The listing builds one solid part. Answer for the finished solid, in the listing's coordinates (mm). A direction names the side the tool comes from. Coordinates: 2 decimals unless noted, no trailing zeros. Loops run counter-clockwise (first coordinate to the right, second up) from the corner with the lowest first, then second, coordinate; pieces in that order, holes last. Notation, with made-up numbers: (-1, 73.25) -> (8, 73.25) arc R11 ccw to (8, 94.25) -> close; hole circle Ø5 at (2.5, 80.25). An arc over 180 degrees is marked (long way). Answer in a Markdown table with one row per item.
```python
from build123d import *

# Parameters (mm, degrees)
F0_W      = 24
F0_H      = 24
F1_DEPTH  = 9.5
F4_R      = 4
F7_DEPTH  = 9.501
F8_DEPTH  = 4.5
F9_DEPTH  = 3.5
F5_R      = 1.35
F10_DEPTH = 9.501


with BuildPart() as f1:
    # F0 (on Top) → F1 (new body)
    with BuildSketch(Plane.XY):
        with Locations((12, 12)):
            Rectangle(F0_W, F0_H)
    extrude(amount=F1_DEPTH)

    # F4
    f4_edges = [f1.edges().sort_by_distance(p)[0] for p in [
        (0, 0, 4.75),
        (24, 0, 4.75),
        (24, 24, 4.75),
        (0, 24, 4.75),
    ]]
    fillet(f4_edges, radius=F4_R)

    # F6 (on face) → F7 (cut, through all)
    with BuildSketch(Plane.XY.offset(9.5)):
        with BuildLine():
            ThreePointArc((15.2, 14.8), (12, 18), (8.8, 14.8))
            Line((8.8, 14.8), (8.8, 9.2))
            ThreePointArc((8.8, 9.2), (12, 6), (15.2, 9.2))
            Line((15.2, 9.2), (15.2, 14.8))
        make_face()
    extrude(amount=-F7_DEPTH, mode=Mode.SUBTRACT)

    # F6 (on face) → F8 (cut, through all)
    with BuildSketch(Plane.XY.offset(9.5)):
        with BuildLine():
            Line((18, 12), (18, 17.291503))
            ThreePointArc((18, 17.291503), (12, 20), (6, 17.291503))
            Line((6, 17.291503), (6, 12))
            Line((6, 12), (6, 6.708497))
            ThreePointArc((6, 6.708497), (12, 4), (18, 6.708497))
            Line((18, 6.708497), (18, 12))
        make_face()
        with BuildLine():
            Line((8.8, 9.2), (8.8, 14.8))
            ThreePointArc((8.8, 14.8), (12, 18), (15.2, 14.8))
            Line((15.2, 14.8), (15.2, 9.2))
            ThreePointArc((15.2, 9.2), (12, 6), (8.8, 9.2))
        make_face(mode=Mode.SUBTRACT)
    extrude(amount=-F8_DEPTH, mode=Mode.SUBTRACT)

    # F6 (on face) → F9 (cut, through all)
    with BuildSketch(Plane.XY.offset(9.5)):
        with BuildLine():
            Line((6, 12), (6, 17.291503))
            ThreePointArc((6, 17.291503), (4, 12), (6, 6.708497))
            Line((6, 6.708497), (6, 12))
        make_face()
        with BuildLine():
            ThreePointArc((18, 6.708497), (19.483315, 9.171573), (20, 12))
            ThreePointArc((20, 12), (19.483315, 14.828427), (18, 17.291503))
            Line((18, 17.291503), (18, 12))
            Line((18, 12), (18, 6.708497))
        make_face()
    extrude(amount=-F9_DEPTH, mode=Mode.SUBTRACT)

    # F5 (on face) → F10 (cut, through all)
    with BuildSketch(Plane.XY.offset(9.5)):
        with Locations((4, 4)):
            Circle(F5_R)
        with Locations((4, 20)):
            Circle(F5_R)
        with Locations((20, 4)):
            Circle(F5_R)
        with Locations((20, 20)):
            Circle(F5_R)
    extrude(amount=-F10_DEPTH, mode=Mode.SUBTRACT)


solid = f1.part
```
Item 1: A cutting plane is placed at A-A, the plane x = 12. Determine the outline of the cut face in (y, z), plus the area to 3 significant figures.
Findings below:
| item | result |
|---|---|
| outline | (0, 0) -> (6, 0) -> (6, 5) -> (4, 5) -> (4, 9.5) -> (0, 9.5) -> close; (18, 0) -> (24, 0) -> (24, 9.5) -> (20, 9.5) -> (20, 5) -> (18, 5) -> close |
| area | 96.0 mm2 |
Item 2: A cutting plane is placed at D-D, the plane y = 3.25. Determine the outline of the cut face in (x, z), plus the area to 3 significant figures.
Findings below:
| item | result |
|---|---|
| outline | (0.07, 0) -> (2.88, 0) -> (2.88, 9.5) -> (0.07, 9.5) -> close; (5.12, 0) -> (18.88, 0) -> (18.88, 9.5) -> (5.12, 9.5) -> close; (21.12, 0) -> (23.93, 0) -> (23.93, 9.5) -> (21.12, 9.5) -> close |
| area | 184 mm2 |
Item 3: Find the intervals of material crossed by probe 1 along X at (y, z) = (13.5, 0.5); probe 2 along Y at (x, z) = (10, 2.5); probe 3 along X at (y, z) = (5, 7.25), in increasing order.
Findings below:
| item | result |
|---|---|
| probe 1 | x = 0 to 8.8, 15.2 to 24 |
| probe 2 | y = 0 to 6.7, 17.3 to 24 |
| probe 3 | x = 0 to 3.09, 4.91 to 8.13, 15.87 to 19.09, 20.91 to 24 |
Item 4: Flat-ended cylindrical pins translate along their axes: pin 1 Ø1.6 at (x, y) = (5, 11) entering from +Z; pin 2 Ø3.5 at (x, y) = (11, 16) entering from +Z; pin 3 Ø1.5 at (y, z) = (21, 5.5) entering from +X. Find the tip coordinate at first contact, or state that the pin passes through.
Findings below:
| item | result |
|---|---|
| pin 1 | stops at z = 6 |
| pin 2 | stops at z = 5 |
| pin 3 | stops at x = 23.99 |
Item 5: A tool of negligible diameter and unlimited length cuts with its end or side. For faces 1 (the face through (15.2, 12, 3)), 2 (the face through (22.797, 1.141, 4.816)), 3 (the face through (8, 12, 5)), from which of +Z, -Z, +X, -X, +Y, -Y can it reach the whole face along a straight path? Write none if from no direction.
Findings below:
| item | result |
|---|---|
| face 1 | +Z, -Z |
| face 2 | +Z, -Z, +X, -Y |
| face 3 | +Z |
Item 6: A cutting plane is placed at C-C, the plane x = 3.5. Determine the outline of the cut face in (y, z).
Findings below:
| item | result |
|---|---|
| outline | (0.03, 0) -> (2.75, 0) -> (2.75, 9.5) -> (0.03, 9.5) -> close; (5.25, 0) -> (18.75, 0) -> (18.75, 9.5) -> (5.25, 9.5) -> close; (21.25, 0) -> (23.97, 0) -> (23.97, 9.5) -> (21.25, 9.5) -> close |
Item 7: A cutting plane is placed at B-B, the plane z = 6.5. Determine the outline of the cut face in (x, y).
Findings below:
| item | result |
|---|---|
| outline | (0, 4) arc R4 ccw to (4, 0) -> (20, 0) arc R4 ccw to (24, 4) -> (24, 20) arc R4 ccw to (20, 24) -> (4, 24) arc R4 ccw to (0, 20) -> close; hole circle Ø2.7 at (4, 4); hole circle Ø2.7 at (4, 20); hole (18, 6.71) arc R8 ccw to (20, 12) arc R8 ccw to (18, 17.29) arc R8 ccw (long way) to start; hole circle Ø2.7 at (20, 4); hole circle Ø2.7 at (20, 20) |
Item 8: Determine the mould class of faces 4 (the face through (12, 24, 5)), 5 (the face through (1.141, 1.203, 4.816)), 6 (the face through (6, 12.1, 5.5)) for opening direction X: +X half, -X half, draft (parallel to the pull), parting line (faces both ways), or undercut.
Findings below:
| item | result |
|---|---|
| face 4 | draft |
| face 5 | -X half |
| face 6 | undercut |
